Verification items for the finished model (mm, model axes). A direction names the side the tool comes from. Give positions to 0.01 mm unless a question says otherwise; leave off trailing zeros. Order: outer loops, then holes, each group sorted by start corner. A loop starts at its lowest first (then second) coordinate and runs counter-clockwise, first axis right, second up. Notation, with made-up numbers: (17, 48.5) - (66, 48.5) arc R15 ccw to (66, 63.5) - close; hole circle Ø1 at (-22, 77). An arc over 180 degrees is marked (long way). Answer as a JSON object with one key per item and string values.
```python
from build123d import *

# Parameters (mm, degrees)
ESQUISSE1_R             = 1.5
BOSS_EXTRU_1_DEPTH      = 5
ENL_V_MAT_EXTRU_1_DEPTH = 10


with BuildPart() as part:
    # Esquisse1 → Boss.-Extru.1 (new body)
    with BuildSketch(Plane.XY):
        with BuildLine():
            Line((14.474115402, 4.43614094), (43.066204977, 20.822692822))
            ThreePointArc((43.066204977, 20.822692822), (67.033056957, 20.765489165), (79, 0))
            ThreePointArc((79, 0), (70, -9), (61, 0))
            ThreePointArc((61, 0), (58.008264239, 5.191372291), (52.016551244, 5.205673206))
            Line((52.016551244, 5.205673206), (23.424461669, -11.180878677))
            ThreePointArc((23.424461669, -11.180878677), (7.285507399, -13.986910655), (-6.894399988, -5.785088487))
            ThreePointArc((-6.894399988, -5.785088487), (-5.785088487, 6.894399988), (6.894399988, 5.785088487))
            ThreePointArc((6.894399988, 5.785088487), (10.439376835, 3.734632945), (14.474115402, 4.43614094))
        make_face()
        with Locations((70, 0)):
            Circle(ESQUISSE1_R, mode=Mode.SUBTRACT)
        Circle(ESQUISSE1_R, mode=Mode.SUBTRACT)
    extrude(amount=BOSS_EXTRU_1_DEPTH)

    # Esquisse2 → Enlèv. mat.-Extru.1 (cut)
    with BuildSketch(Plane.XY.offset(5)):
        with BuildLine():
            ThreePointArc((4.401541671, -13.287300689), (18.082976377, -6.617066031), (33.265702076, -5.540717398))
            ThreePointArc((33.265702076, -5.540717398), (20.118574556, -14.201807608), (4.401541671, -13.287300689))
        make_face()
    extrude(amount=-ENL_V_MAT_EXTRU_1_DEPTH, mode=Mode.SUBTRACT)


solid = part.part
```
(1) Gauge pin test, flat ends, axial feed: pin 1 Ø2.5 at (x, y) = (0, 0) entering from +Z; pin 2 Ø1.5 at (x, y) = (40.5, 11.5) entering from -Z; pin 3 Ø2 at (x, z) = (35, 3.5) entering from +Y. Record the tip position at first contact, or that the pin passes through.
Computed values:
{"pin 1": "passes through", "pin 2": "stops at z = 0", "pin 3": "stops at y = 16.77"}
(2) Release check for a two-part mould opening along X. For faces 4 (the cylindrical face through (17.876, -6.673, 2.535)), 5 (the cylindrical face through (-1.71, -10.4, 2.46)), 6 (the flat face through (36, 6, 0)) record: pulls with the +X half, pulls with the -X half, needs draft (parallel to the pull), parting line crosses it, or undercut.
Computed values:
{"face 4": "undercut", "face 5": "pulls with the -X half", "face 6": "needs draft"}
(3) Material ranges on line 1 along Y through (x, z) = (70, 3.65) (3 decimals); line 2 along X through (y, z) = (2, 0.4); line 3 along X through (y, z) = (3.5, 4.55), recorded low to high. Write a range as [from, to].
Computed values:
{"line 1": "y = [-9, -1.5], [1.5, 18.735]", "line 2": "x = [-8.77, 46.42], [60.66, 78.92]", "line 3": "x = [-8.29, 49.04], [59.87, 78.74]"}
(4) Access from +Z, -Z, +X, -X, +Y, -Y to the whole of each face (thin tool, end or side, straight path). Record for faces 1 (the cylindrical face through (-1.5, 0.07, 2.46)), 2 (the flat face through (28.57, 12.515, 2.465)), 3 (the flat face through (42.772, -0.092, 2.465)).
Computed values:
{"face 1": "+Z, -Z", "face 2": "+Z, -Z, +Y", "face 3": "+Z, -Z, -Y"}
(5) Section check C-C (x = 0). Record the cut outline in (y, z), then the cut area to 3 significant figures.
Computed values:
{"outline": "(-11.43, 0) - (-1.5, 0) - (-1.5, 5) - (-11.43, 5) - close; (1.5, 0) - (9, 0) - (9, 5) - (1.5, 5) - close", "area": "87.1 mm²"}
(6) Section check B-B (z = 4.15). Record the cut outline in (x, y), then the cut area to 3 significant figures.
Computed values:
{"outline": "(-6.89, -5.79) arc R24 ccw to (4.4, -13.29) arc R40 cw to (33.27, -5.54) - (52.02, 5.21) arc R6 cw to (61, 0) arc R9 ccw to (79, 0) arc R24 ccw to (43.07, 20.82) - (14.47, 4.44) arc R6 cw to (6.89, 5.79) arc R9 ccw to start; hole circle Ø3 at (0, 0); hole circle Ø3 at (70, 0)", "area": "1,650 mm²"}
(7) Section check A-A (x = 70). Record the cut outline in (y, z) (3 decimals).
Computed values:
{"outline": "(-9, 0) - (-1.5, 0) - (-1.5, 5) - (-9, 5) - close; (1.5, 0) - (18.735, 0) - (18.735, 5) - (1.5, 5) - close"}
(8) Section check D-D (y = -10). Record the cut outline in (x, z).
Computed values:
{"outline": "(-2.3, 0) - (9.55, 0) - (9.55, 5) - (-2.3, 5) - close"}
